from build123d import *

# Parameters (mm, degrees)
F2_R     = 4.7625
F3_DEPTH = 9.525
F4_R     = 1.5875
F5_DEPTH = 16.66875
F6_DEPTH = 25.4


with BuildPart() as f1:
    # F0 (on Front) → F1 (revolve)
    with BuildSketch(Plane.XZ):
        with BuildLine():
            Line((0, 50.8), (0, 0))
            Line((0, 0), (10.2612478659, 0))
            Line((10.2612478659, 0), (21.9292579814, 7.1549119122))
            ThreePointArc((21.9292579814, 7.1549119122), (24.1505997169, 9.4662699385), (24.9597914517, 12.5681957545))
            Line((24.9597914517, 12.5681957545), (24.9597914517, 17.3331890255))
            Line((24.9597914517, 17.3331890255), (10.2612478659, 17.3331890255))
            Line((10.2612478659, 17.3331890255), (10.2612478659, 50.8))
            Line((10.2612478659, 50.8), (0, 50.8))
        make_face()
    revolve(axis=Axis((0, 0, 25.4), (0, 0, 1)))

    # F2 (on face) → F3 (cut)
    with BuildSketch(Plane.XY.offset(50.8)):
        Circle(F2_R)
    extrude(amount=-F3_DEPTH, mode=Mode.SUBTRACT)

    # F4 (on face) → F5 (cut)
    with BuildSketch(Plane(origin=(0, 0, 0), x_dir=(1, 0, 0), z_dir=(0, 0, -1))):
        Circle(F4_R)
    extrude(amount=-F5_DEPTH, mode=Mode.SUBTRACT)

    # F6 (add): a face of the model
    f6_faces = [f1.faces().sort_by_distance(p)[0] for p in [
        (-24.25382194, 0, 17.3331890255),
    ]]
    extrude(f6_faces, amount=F6_DEPTH)


solid = f1.part
Build history of the part. All positions in model axes, mm. A direction names the side the tool comes from. Round coordinates to 2 decimals unless told otherwise and drop trailing zeros. Write each loop counter-clockwise with the first axis right and the second up, starting at its lowest first coordinate (ties: lowest second). Pieces come first, ordered by that corner, then holes. Notation, with made-up numbers: (-19, 37) -> (-7, 37) arc R10 ccw to (-7, 47) -> close; hole circle Ø6 at (-14, 25). An arc over 180 degrees is marked (long way). Use one line per item in the form item = value.
Q1. Drill centre lines: L1, parallel to Y at x = 0, z = 5; L2, parallel to Y at x = 0, z = 11; L3, parallel to Z at x = -4.5, y = 0.5 (3 decimals). Where is each one in solid material? Low to high.
Conclusion:
L1 = -18.42 to -1.59, 1.59 to 18.42
L2 = -24.76 to -1.59, 1.59 to 24.76
L3 = 0 to 41.275
Q2. Drop flat-ended pins along their axis: P1, Ø2.5, axis at x = 0.5, y = -1, coming from the -Z side; P2, Ø5, axis at x = -9.5, y = -16.5, coming from the +Z side; P3, Ø1.5, axis at y = -7, z = 16.5, coming from the -X side; P4, Ø6, axis at y = -15.5, z = 43, coming from the +X side. Give the stop position or say it passes through.
Conclusion:
P1 = 0
P2 = 42.73
P3 = -24.16
P4 = 21.6
Q3. Band-saw the part on D-D, the plane z = 45.5. Write the cut outline in (x, y) (1 decimal), then the cut area to 3 significant figures.
Conclusion:
outline = circle Ø20.5 at (0, 0); hole circle Ø9.5 at (0, 0)
area = 260 mm²
Q4. Band-saw the part on C-C, the plane z = 23.5. Write the cut outline in (x, y).
Conclusion:
outline = circle Ø49.92 at (0, 0)
Q5. Tool access for faces 1 (the flat face through (0, 0, 16.669)), 2 (the cylindrical face through (-3.78, -2.9, 46.1)), 3 (the flat face through (4.4, 2.4, 50.8)): list every direction of +Z, -Z, +X, -X, +Y, -Y with a clear straight run to the whole face (end or side of a thin tool).
Conclusion:
face_1 = -Z
face_2 = +Z
face_3 = +Z, +X, -X, +Y, -Y
